Input: part model. Units: mm. Frame: model coordinates. Coordinates: 2 decimals unless noted, no trailing zeros. Write each loop counter-clockwise with the first axis right and the second up, starting at its lowest first coordinate (ties: lowest second). Pieces come first, ordered by that corner, then holes. Notation, with made-up numbers: M 64.5,36 L 88.5,36 A25 ccw 88.5,52 Z; hole C -19.5,-31.5 d4. An arc over 180 degrees is marked long. Use CSV: the item, a comma, the result in double quotes.
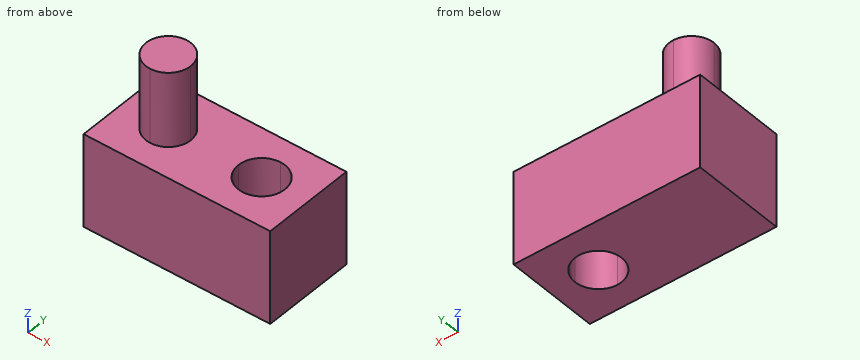
```python
from build123d import *

# Parameters (mm, degrees)
F1_DEPTH = 12.7
F3_DEPTH = 10.16


with BuildPart() as f1:
    # F0 (on Top) → F1 (new body)
    with BuildSketch(Plane.XY):
        with BuildLine():
            Line((-6.35, -6.35), (6.35, -6.35))
            Line((6.35, -6.35), (6.35, -3.175))
            ThreePointArc((6.35, -3.175), (4.1049359697, -2.2450640303), (3.175, 0))
            Line((3.175, 0), (-3.302, 0))
            ThreePointArc((-3.302, 0), (-4.1947385309, -2.1552614691), (-6.35, -3.048))
            Line((-6.35, -3.048), (-6.35, -6.35))
        make_face()
        with BuildLine():
            Line((-3.302, 0), (3.175, 0))
            ThreePointArc((3.175, 0), (4.1049359697, 2.2450640303), (6.35, 3.175))
            Line((6.35, 3.175), (6.35, 6.35))
            Line((6.35, 6.35), (-6.35, 6.35))
            Line((-6.35, 6.35), (-6.35, 3.048))
            ThreePointArc((-6.35, 3.048), (-4.1947385309, 2.1552614691), (-3.302, 0))
        make_face()
        with BuildLine():
            Line((9.525, 0), (12.7, 0))
            Line((12.7, 0), (12.7, 6.35))
            Line((12.7, 6.35), (6.35, 6.35))
            Line((6.35, 6.35), (6.35, 3.175))
            ThreePointArc((6.35, 3.175), (8.5950640303, 2.2450640303), (9.525, 0))
        make_face()
        with BuildLine():
            Line((6.35, -6.35), (12.7, -6.35))
            Line((12.7, -6.35), (12.7, 0))
            Line((12.7, 0), (9.525, 0))
            ThreePointArc((9.525, 0), (8.5950640303, -2.2450640303), (6.35, -3.175))
            Line((6.35, -3.175), (6.35, -6.35))
        make_face()
        with BuildLine():
            Line((-12.7, -6.35), (-6.35, -6.35))
            Line((-6.35, -6.35), (-6.35, -3.048))
            ThreePointArc((-6.35, -3.048), (-8.5052614691, -2.1552614691), (-9.398, 0))
            Line((-9.398, 0), (-12.7, 0))
            Line((-12.7, 0), (-12.7, -6.35))
        make_face()
        with BuildLine():
            Line((-12.7, 6.35), (-12.7, 0))
            Line((-12.7, 0), (-9.398, 0))
            ThreePointArc((-9.398, 0), (-8.5052614691, 2.1552614691), (-6.35, 3.048))
            Line((-6.35, 3.048), (-6.35, 6.35))
            Line((-6.35, 6.35), (-12.7, 6.35))
        make_face()
        with BuildLine():
            Line((-6.35, 3.048), (-6.35, 0))
            Line((-6.35, 0), (-3.302, 0))
            ThreePointArc((-3.302, 0), (-4.1947385309, 2.1552614691), (-6.35, 3.048))
        make_face()
        with BuildLine():
            Line((-9.398, 0), (-6.35, 0))
            Line((-6.35, 0), (-6.35, 3.048))
            ThreePointArc((-6.35, 3.048), (-8.5052614691, 2.1552614691), (-9.398, 0))
        make_face()
        with BuildLine():
            ThreePointArc((-9.398, 0), (-8.5052614691, -2.1552614691), (-6.35, -3.048))
            Line((-6.35, -3.048), (-6.35, 0))
            Line((-6.35, 0), (-9.398, 0))
        make_face()
        with BuildLine():
            Line((-6.35, 0), (-6.35, -3.048))
            ThreePointArc((-6.35, -3.048), (-4.1947385309, -2.1552614691), (-3.302, 0))
            Line((-3.302, 0), (-6.35, 0))
        make_face()
    extrude(amount=F1_DEPTH)

    # F2 (on face) → F3 (join)
    with BuildSketch(Plane.XY.offset(12.7)):
        with BuildLine():
            Line((-6.35, 0), (-6.35, -3.048))
            ThreePointArc((-6.35, -3.048), (-4.1947385309, -2.1552614691), (-3.302, 0))
            Line((-3.302, 0), (-6.35, 0))
        make_face()
        with BuildLine():
            Line((-6.35, 3.048), (-6.35, 0))
            Line((-6.35, 0), (-3.302, 0))
            ThreePointArc((-3.302, 0), (-4.1947385309, 2.1552614691), (-6.35, 3.048))
        make_face()
        with BuildLine():
            ThreePointArc((-9.398, 0), (-8.5052614691, -2.1552614691), (-6.35, -3.048))
            Line((-6.35, -3.048), (-6.35, 0))
            Line((-6.35, 0), (-9.398, 0))
        make_face()
        with BuildLine():
            Line((-9.398, 0), (-6.35, 0))
            Line((-6.35, 0), (-6.35, 3.048))
            ThreePointArc((-6.35, 3.048), (-8.5052614691, 2.1552614691), (-9.398, 0))
        make_face()
    extrude(amount=F3_DEPTH)


solid = f1.part
```
1. Section D-D (z = 19.5). Return loops of the section in (x, y).
Resolved:
outline,"C -6.35,0 d6.1"
2. Material intervals for line 1 (Z direction, x = 9.25, y = 4.5); line 2 (Y direction, x = 5.5, z = 10.75); line 3 (X direction, y = 2.25, z = 5), sorted ascending. Write a range as [from, to].
Resolved:
line 1,"z = [0, 12.7]"
line 2,"y = [-6.35, -3.06], [3.06, 6.35]"
line 3,"x = [-12.7, 4.11], [8.59, 12.7]"
3. Section B-B (y = -1). Return loops of the section in (x, z).
Resolved:
outline,"M -12.7,0 L 3.34,0 L 3.34,12.7 L -3.47,12.7 L -3.47,22.86 L -9.23,22.86 L -9.23,12.7 L -12.7,12.7 Z; M 9.36,0 L 12.7,0 L 12.7,12.7 L 9.36,12.7 Z"
4. Section A-A (z = 8). Return loops of the section in (x, y) (3 decimals), then the cut area to 3 significant figures.
Resolved:
outline,"M -12.7,-6.35 L 12.7,-6.35 L 12.7,6.35 L -12.7,6.35 Z; hole C 6.35,0 d6.35"
area,"291 mm^2"
5. Section C-C (x = -4.25). Return loops of the section in (y, z), then the cut area to 3 significant figures.
Resolved:
outline,"M -6.35,0 L 6.35,0 L 6.35,12.7 L 2.21,12.7 L 2.21,22.86 L -2.21,22.86 L -2.21,12.7 L -6.35,12.7 Z"
area,"206 mm^2"
